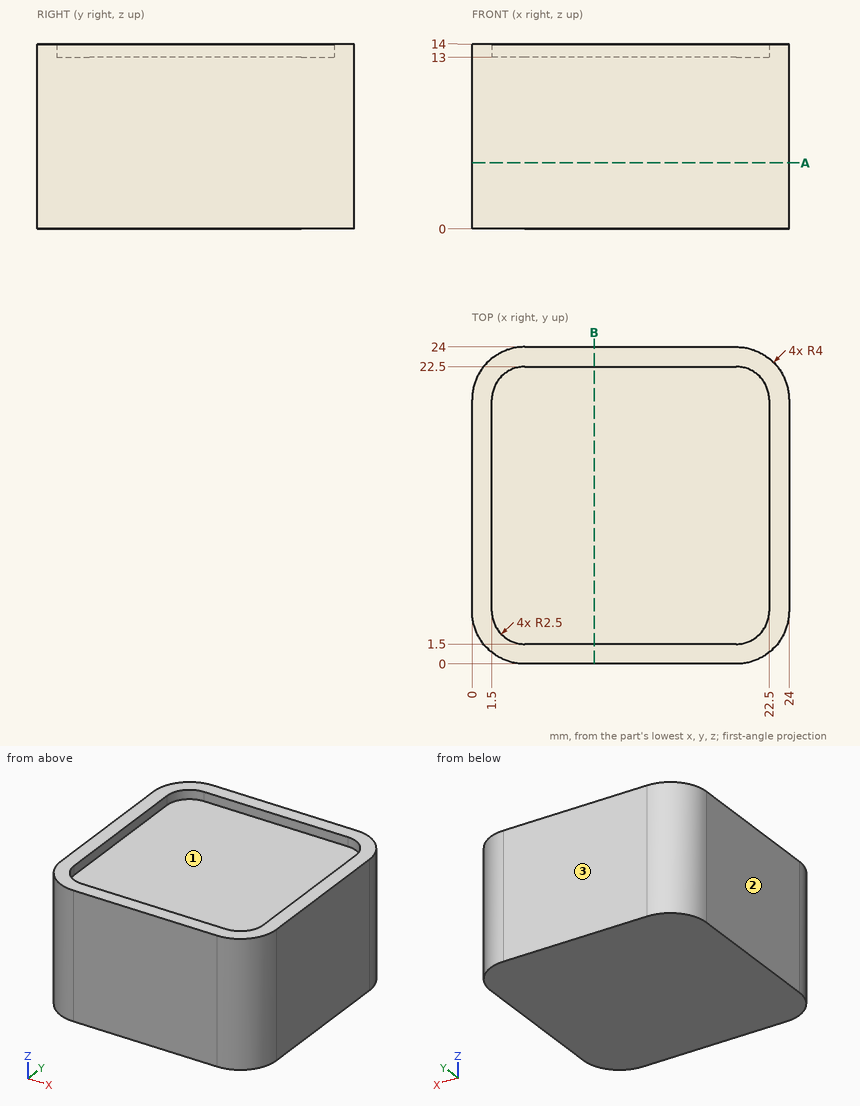
Part print with two shaded views. Sizes in mm from the minimum x, y, z corner. Round coordinates to 2 decimals unless told otherwise and drop trailing zeros. Order: outer loops, then holes, each group sorted by start corner. A loop starts at its lowest first (then second) coordinate and runs counter-clockwise, first axis right, second up. Notation, with made-up numbers: (-4.75, 26.5) -> (7.25, 26.5) arc R4 cw to (7.25, 33.5) -> close; hole circle Ø6 at (-38.75, 37.5). An arc over 180 degrees is marked (long way). One line per question, with ' | ' between items.
Q1. Slice it at B-B (x = 9.25). Write the cut outline in (y, z).
Completed:
outline: (0, 0) -> (24, 0) -> (24, 14) -> (22.5, 14) -> (22.5, 13) -> (1.5, 13) -> (1.5, 14) -> (0, 14) -> close
Q2. Probe probe 1 along Z at (x, y) = (14.5, 22.25); probe 2 along X at (y, z) = (2.5, 8.5); probe 3 along Y at (x, z) = (1.25, 6.25). List the from-to ranges inside material, lowest first.
Completed:
probe 1: z = 0 to 13 | probe 2: x = 0.29 to 23.71 | probe 3: y = 1.1 to 22.9
Q3. Drop flat-ended pins along their axis: pin 1 (6.5 mm diameter, centred on x = 9.5, y = 7, fed in from +Z); pin 2 (1.5 mm diameter, centred on y = 12.5, z = 7.5, fed in from -X). Give the stop position or say it passes through.
Completed:
pin 1: stops at z = 13 | pin 2: stops at x = 0
Q4. Slice it at A-A (z = 5). Write the cut outline in (x, y).
Completed:
outline: (0, 4) arc R4 ccw to (4, 0) -> (20, 0) arc R4 ccw to (24, 4) -> (24, 20) arc R4 ccw to (20, 24) -> (4, 24) arc R4 ccw to (0, 20) -> close
Q5. Two-plate mould, pull along Y, no slides. Class the marked faces 1, 2 and 3: released by +Y, released by -Y, zero draft, split by the parting line, or undercut.
Completed:
face 1: undercut | face 2: zero draft | face 3: released by +Y
